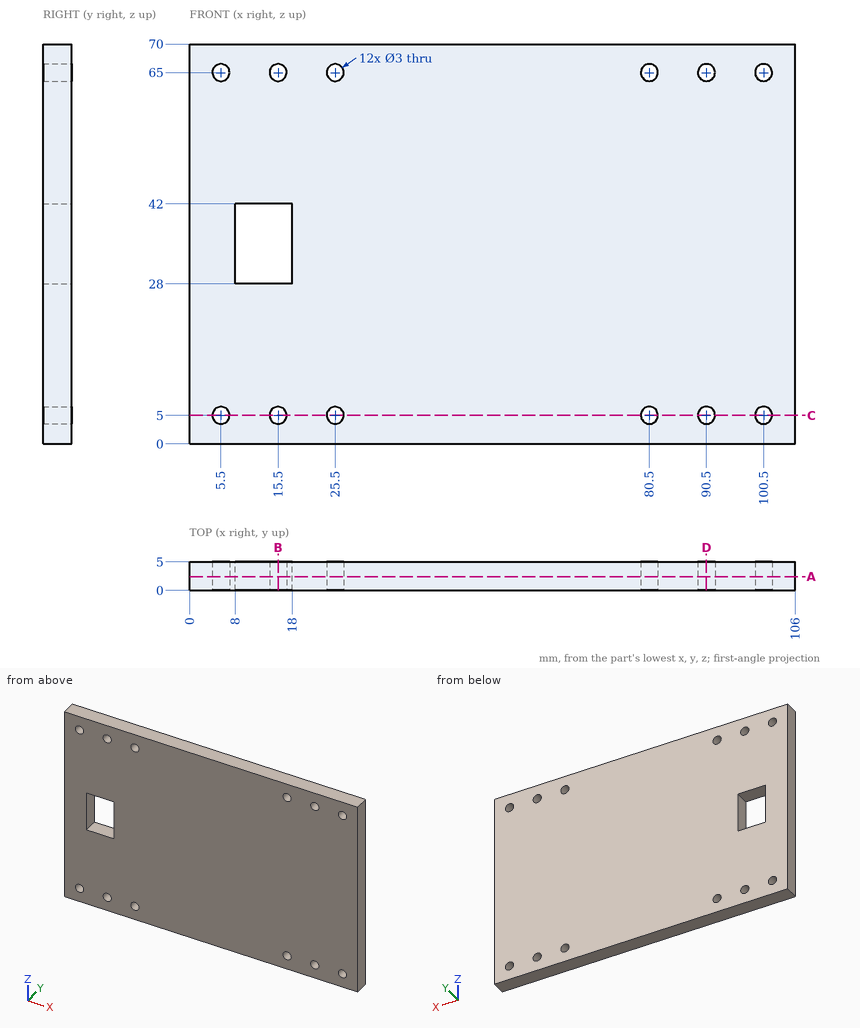
Could you check a few things on this drawing? It's one solid part, dimensions in mm from its lowest x, y, z. Give positions to 0.01 mm unless a question says otherwise; leave off trailing zeros. Write each loop counter-clockwise with the first axis right and the second up, starting at its lowest first coordinate (ties: lowest second). Pieces come first, ordered by that corner, then holes. Notation, with made-up numbers: M 3,-24.75 L 42,-24.75 A23 ccw 42,-16.75 Z; hole C -25.75,36 d4. An arc over 180 degrees is marked long. Put each result on its own line as item: value. Start each with the question number.
Item 1: I need wall thicknesses on L1, parallel to Z at x = 100.5, y = 3.55; L2, parallel to X at y = 3.8, z = 40. Which ranges of each line are inside material? Lowest first, please. Write a range as from..to.
Item 2: If we section it at D-D, the plane x = 90.5: Write out the boundary of the cut face in (y, z).
Item 3: If we section it at A-A, the plane y = 2.4: Count the separate pieces of the cut face and the enclosed holes in it, then the cut area to 3 significant figures.
Item 4: If we section it at C-C, the plane z = 5: Write out the boundary of the cut face in (x, y), then the cut area to 3 significant figures.
Item 5: If we section it at B-B, the plane x = 15.5: Write out the boundary of the cut face in (y, z).
Values:
1. L1: 0..3.5, 6.5..63.5, 66.5..70
1. L2: 0..8, 18..106
2. outline: M 0,0 L 5,0 L 5,3.5 L 0,3.5 Z; M 0,6.5 L 5,6.5 L 5,63.5 L 0,63.5 Z; M 0,66.5 L 5,66.5 L 5,70 L 0,70 Z
3. separate pieces: 1
3. enclosed holes: 13
3. area: 7,200 mm²
4. outline: M 0,0 L 4,0 L 4,5 L 0,5 Z; M 7,0 L 14,0 L 14,5 L 7,5 Z; M 17,0 L 24,0 L 24,5 L 17,5 Z; M 27,0 L 79,0 L 79,5 L 27,5 Z; M 82,0 L 89,0 L 89,5 L 82,5 Z; M 92,0 L 99,0 L 99,5 L 92,5 Z; M 102,0 L 106,0 L 106,5 L 102,5 Z
4. area: 440 mm²
5. outline: M 0,0 L 5,0 L 5,3.5 L 0,3.5 Z; M 0,6.5 L 5,6.5 L 5,28 L 0,28 Z; M 0,42 L 5,42 L 5,63.5 L 0,63.5 Z; M 0,66.5 L 5,66.5 L 5,70 L 0,70 Z
